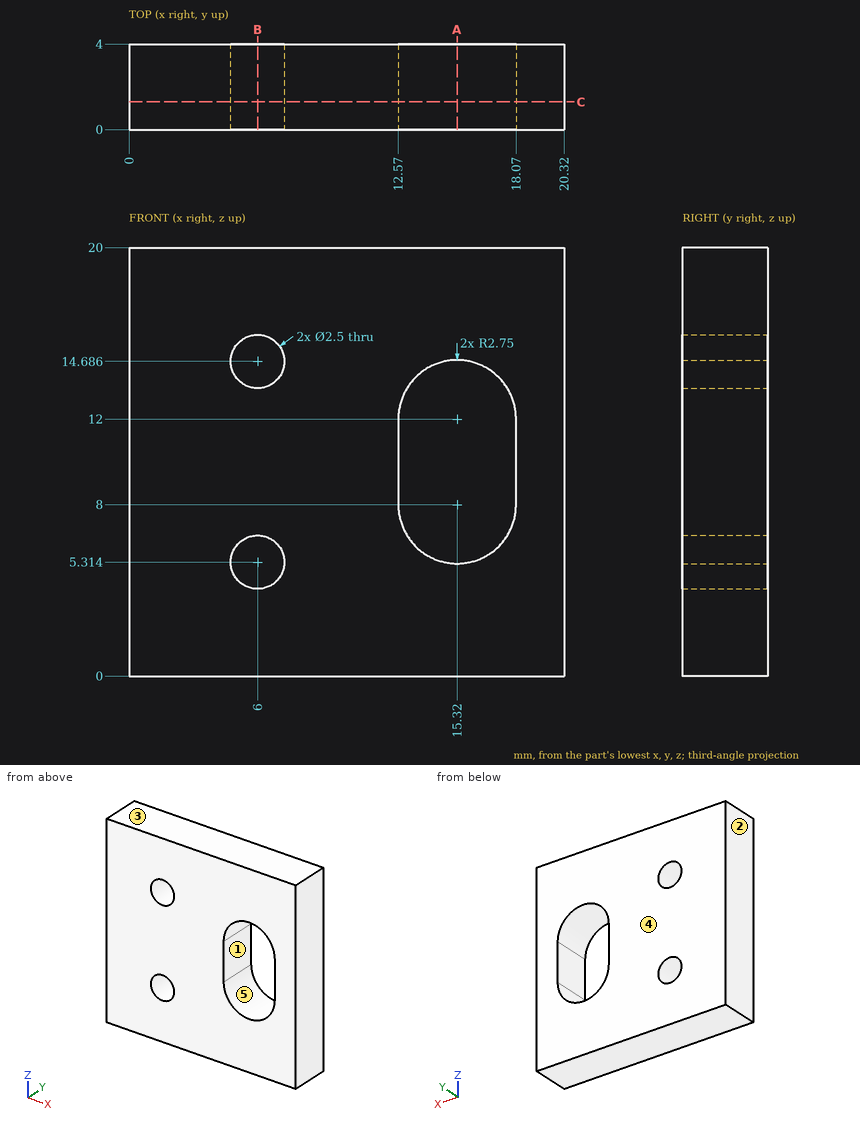
Input: dimensioned drawing with shaded views. Units: mm. Origin: part minimum x, y, z. A direction names the side the tool comes from. Coordinates: 2 decimals unless noted, no trailing zeros. Write each loop counter-clockwise with the first axis right and the second up, starting at its lowest first coordinate (ties: lowest second). Pieces come first, ordered by that corner, then holes. Notation, with made-up numbers: M -32,-33 L 25,-33 A23 cw 25,4 Z; hole C 61.25,-1.75 d8. An arc over 180 degrees is marked long. Answer as CSV lines item,"result". Start each with the question number.
Q1. Cut plane C-C on y = 1.3. Return the cut outline in (x, z).
Q2. Reachability of the marked faces 1 and 2 from +Z, -Z, +X, -X, +Y, -Y: full face, straight path, thin tool, end or side. Return the list, or none.
Q3. Cut plane A-A on x = 15.32. Return the cut outline in (y, z).
Q4. Mould query, pull axis Z, two halves, no side actions, for the marked faces 3, 4 and 5. Classes: released by +Z, released by -Z, zero draft, split by the parting line, or undercut.
Q5. Cut plane B-B on x = 6. Return the cut outline in (y, z).
Q6. Line query: line 1 (Z direction, x = 6, y = 0.9); line 2 (X direction, y = 2.4, z = 8); line 3 (Z direction, x = 5, y = 1.65). Output: solid intervals per line, ascending. Write a range as from..to.
Findings below:
1,outline,"M 0,0 L 20.32,0 L 20.32,20 L 0,20 Z; hole C 6,5.31 d2.5; hole C 6,14.69 d2.5; hole M 12.57,8 A2.75 ccw 18.07,8 L 18.07,12 A2.75 ccw 12.57,12 Z"
2,face 1,"+Y, -Y"
2,face 2,"+Z, -Z, -X, +Y, -Y"
3,outline,"M 0,0 L 4,0 L 4,5.25 L 0,5.25 Z; M 0,14.75 L 4,14.75 L 4,20 L 0,20 Z"
4,face 3,"released by +Z"
4,face 4,"zero draft"
4,face 5,"undercut"
5,outline,"M 0,0 L 4,0 L 4,4.06 L 0,4.06 Z; M 0,6.56 L 4,6.56 L 4,13.44 L 0,13.44 Z; M 0,15.94 L 4,15.94 L 4,20 L 0,20 Z"
6,line 1,"z = 0..4.06, 6.56..13.44, 15.94..20"
6,line 2,"x = 0..12.57, 18.07..20.32"
6,line 3,"z = 0..4.56, 6.06..13.94, 15.44..20"
